Geometry: see drawing. Coordinates: mm, zero at the bounding-box minimum. A direction names the side the tool comes from. Round coordinates to 2 decimals unless told otherwise and drop trailing zeros. Write each loop counter-clockwise with the first axis right and the second up, starting at its lowest first coordinate (ties: lowest second). Pieces come first, ordered by that corner, then holes.
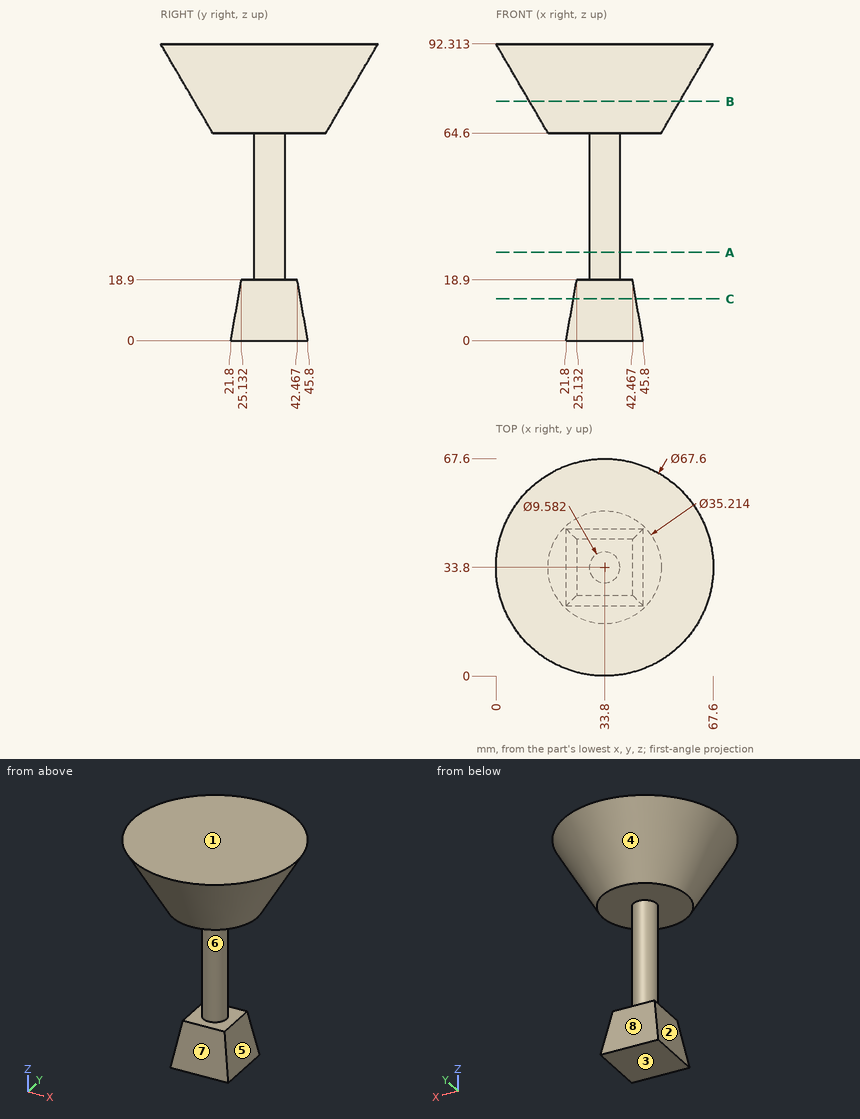
1) Section query C-C on z = 13. Return the cut outline in (x, y).
Taken from the geometry:
outline: (24.09, 24.09) - (43.51, 24.09) - (43.51, 43.51) - (24.09, 43.51) - close
2) Pull-direction query (Z, two-part tool) for the marked faces 1, 2 and 3; classes: released by +Z, released by -Z, zero draft, split by the parting line, or undercut.
Taken from the geometry:
face 1: released by +Z
face 2: undercut
face 3: released by -Z
3) Section query B-B on z = 74.5. Return the cut outline in (x, y), then the cut area to 3 significant figures.
Taken from the geometry:
outline: circle Ø46.78 at (33.8, 33.8)
area: 1,720 mm2
4) Reachability of the marked faces 4, 5, 6, 7 and 8 from +Z, -Z, +X, -X, +Y, -Y: full face, straight path, thin tool, end or side. Return the list, or none.
Taken from the geometry:
face 4: -Z
face 5: +X, +Y, -Y
face 6: none
face 7: +X, -X, -Y
face 8: +X, -X, +Y
5) Material intervals for line 1 (Z direction, x = 36, y = 28.5); line 2 (Z direction, x = 19.5, y = 34); line 3 (Y direction, x = 34, z = 23), sorted ascending.
Taken from the geometry:
line 1: z = 0 to 18.9, 64.6 to 92.31
line 2: z = 64.6 to 92.31
line 3: y = 29.01 to 38.59
6) Contact query for flat-ended pins moving along their axis: P1, Ø5, axis at x = 56, y = 51.5, coming from the -Z side; P2, Ø1, axis at x = 7.5, y = 21, coming from the -Z side; P3, Ø10, axis at y = 43.5, z = 19.5, coming from the +X side. Output: stop coordinate, or through.
Taken from the geometry:
P1: stops at z = 78.78
P2: stops at z = 83.67
P3: stops at x = 43.24
7) Section query A-A on z = 27.5. Return the cut outline in (x, y), then the cut area to 3 significant figures.
Taken from the geometry:
outline: circle Ø9.58 at (33.8, 33.8)
area: 72.1 mm2
